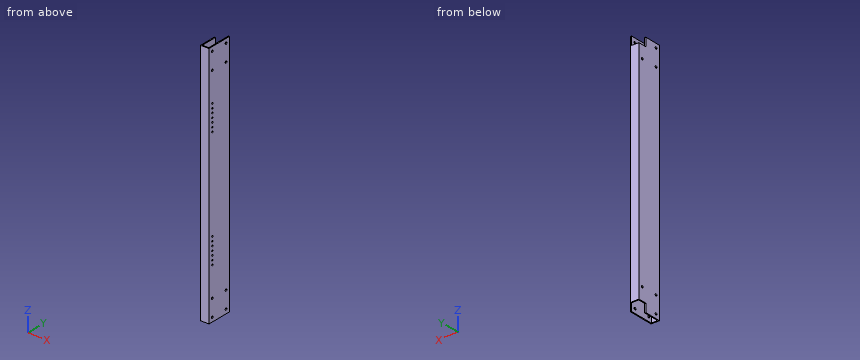
```python
from build123d import *

# Parameters (mm, degrees)
SKETCH1_W               = 25.4
SKETCH1_H               = 76.2
BOSS_EXTRUDE1_DEPTH     = 368.3
SHELL1_T                = -3.175
CUT_EXTRUDE2_REACH      = 27.4
SKETCH3_R               = 2.38125
SKETCH4_W               = 25.4
SKETCH4_H               = 25.4
CUT_EXTRUDE3_DEPTH      = 22.225
SKETCH5_R               = 3.25
CUT_EXTRUDE4_DEPTH      = 23.225
CUT_EXTRUDE4_DEPTH_BACK = 4.175


with BuildPart() as part:
    # Sketch1 → Boss-Extrude1 (new body, symmetric)
    with BuildSketch(Plane.XY):
        Rectangle(SKETCH1_W, SKETCH1_H)
    extrude(amount=BOSS_EXTRUDE1_DEPTH, both=True)

    # Shell1
    shell1_openings = [part.faces().sort_by_distance(p)[0] for p in [
        (0, 0, 368.3),
        (0, 0, -368.3),
    ]]
    offset(amount=SHELL1_T, openings=shell1_openings, kind=Kind.INTERSECTION)

    # Sketch3 → Cut-Extrude2 (cut, up to next)
    with BuildSketch(Plane(origin=(12.7, 0, 0), x_dir=(0, 0, -1), z_dir=(1, 0, 0)), mode=Mode.PRIVATE) as cut_extrude2_sk1:
        with Locations((215.9, -25.4)):
            Circle(SKETCH3_R)
    cut_extrude2_tool1 = extrude(cut_extrude2_sk1.sketch, amount=-CUT_EXTRUDE2_REACH, mode=Mode.PRIVATE) & part.part
    add(cut_extrude2_tool1.solids().sort_by_distance((12.7, -25.4, -215.9))[0], mode=Mode.SUBTRACT)
    # Sketch3 → Cut-Extrude2 (cut, up to next)
    with BuildSketch(Plane(origin=(12.7, 0, 0), x_dir=(0, 0, -1), z_dir=(1, 0, 0)), mode=Mode.PRIVATE) as cut_extrude2_sk2:
        with Locations((203.2, -25.4)):
            Circle(SKETCH3_R)
    cut_extrude2_tool2 = extrude(cut_extrude2_sk2.sketch, amount=-CUT_EXTRUDE2_REACH, mode=Mode.PRIVATE) & part.part
    add(cut_extrude2_tool2.solids().sort_by_distance((12.7, -25.4, -203.2))[0], mode=Mode.SUBTRACT)
    # Sketch3 → Cut-Extrude2 (cut, up to next)
    with BuildSketch(Plane(origin=(12.7, 0, 0), x_dir=(0, 0, -1), z_dir=(1, 0, 0)), mode=Mode.PRIVATE) as cut_extrude2_sk3:
        with Locations((190.5, -25.4)):
            Circle(SKETCH3_R)
    cut_extrude2_tool3 = extrude(cut_extrude2_sk3.sketch, amount=-CUT_EXTRUDE2_REACH, mode=Mode.PRIVATE) & part.part
    add(cut_extrude2_tool3.solids().sort_by_distance((12.7, -25.4, -190.5))[0], mode=Mode.SUBTRACT)
    # Sketch3 → Cut-Extrude2 (cut, up to next)
    with BuildSketch(Plane(origin=(12.7, 0, 0), x_dir=(0, 0, -1), z_dir=(1, 0, 0)), mode=Mode.PRIVATE) as cut_extrude2_sk4:
        with Locations((177.8, -25.4)):
            Circle(SKETCH3_R)
    cut_extrude2_tool4 = extrude(cut_extrude2_sk4.sketch, amount=-CUT_EXTRUDE2_REACH, mode=Mode.PRIVATE) & part.part
    add(cut_extrude2_tool4.solids().sort_by_distance((12.7, -25.4, -177.8))[0], mode=Mode.SUBTRACT)
    # Sketch3 → Cut-Extrude2 (cut, up to next)
    with BuildSketch(Plane(origin=(12.7, 0, 0), x_dir=(0, 0, -1), z_dir=(1, 0, 0)), mode=Mode.PRIVATE) as cut_extrude2_sk5:
        with Locations((165.1, -25.4)):
            Circle(SKETCH3_R)
    cut_extrude2_tool5 = extrude(cut_extrude2_sk5.sketch, amount=-CUT_EXTRUDE2_REACH, mode=Mode.PRIVATE) & part.part
    add(cut_extrude2_tool5.solids().sort_by_distance((12.7, -25.4, -165.1))[0], mode=Mode.SUBTRACT)
    # Sketch3 → Cut-Extrude2 (cut, up to next)
    with BuildSketch(Plane(origin=(12.7, 0, 0), x_dir=(0, 0, -1), z_dir=(1, 0, 0)), mode=Mode.PRIVATE) as cut_extrude2_sk6:
        with Locations((152.4, -25.4)):
            Circle(SKETCH3_R)
    cut_extrude2_tool6 = extrude(cut_extrude2_sk6.sketch, amount=-CUT_EXTRUDE2_REACH, mode=Mode.PRIVATE) & part.part
    add(cut_extrude2_tool6.solids().sort_by_distance((12.7, -25.4, -152.4))[0], mode=Mode.SUBTRACT)
    # Sketch3 → Cut-Extrude2 (cut, up to next)
    with BuildSketch(Plane(origin=(12.7, 0, 0), x_dir=(0, 0, -1), z_dir=(1, 0, 0)), mode=Mode.PRIVATE) as cut_extrude2_sk7:
        with Locations((139.7, -25.4)):
            Circle(SKETCH3_R)
    cut_extrude2_tool7 = extrude(cut_extrude2_sk7.sketch, amount=-CUT_EXTRUDE2_REACH, mode=Mode.PRIVATE) & part.part
    add(cut_extrude2_tool7.solids().sort_by_distance((12.7, -25.4, -139.7))[0], mode=Mode.SUBTRACT)
    # Sketch3 → Cut-Extrude2 (cut, up to next)
    with BuildSketch(Plane(origin=(12.7, 0, 0), x_dir=(0, 0, -1), z_dir=(1, 0, 0)), mode=Mode.PRIVATE) as cut_extrude2_sk8:
        with Locations((-139.7, -25.4)):
            Circle(SKETCH3_R)
    cut_extrude2_tool8 = extrude(cut_extrude2_sk8.sketch, amount=-CUT_EXTRUDE2_REACH, mode=Mode.PRIVATE) & part.part
    add(cut_extrude2_tool8.solids().sort_by_distance((12.7, -25.4, 139.7))[0], mode=Mode.SUBTRACT)
    # Sketch3 → Cut-Extrude2 (cut, up to next)
    with BuildSketch(Plane(origin=(12.7, 0, 0), x_dir=(0, 0, -1), z_dir=(1, 0, 0)), mode=Mode.PRIVATE) as cut_extrude2_sk9:
        with Locations((-152.4, -25.4)):
            Circle(SKETCH3_R)
    cut_extrude2_tool9 = extrude(cut_extrude2_sk9.sketch, amount=-CUT_EXTRUDE2_REACH, mode=Mode.PRIVATE) & part.part
    add(cut_extrude2_tool9.solids().sort_by_distance((12.7, -25.4, 152.4))[0], mode=Mode.SUBTRACT)
    # Sketch3 → Cut-Extrude2 (cut, up to next)
    with BuildSketch(Plane(origin=(12.7, 0, 0), x_dir=(0, 0, -1), z_dir=(1, 0, 0)), mode=Mode.PRIVATE) as cut_extrude2_sk10:
        with Locations((-165.1, -25.4)):
            Circle(SKETCH3_R)
    cut_extrude2_tool10 = extrude(cut_extrude2_sk10.sketch, amount=-CUT_EXTRUDE2_REACH, mode=Mode.PRIVATE) & part.part
    add(cut_extrude2_tool10.solids().sort_by_distance((12.7, -25.4, 165.1))[0], mode=Mode.SUBTRACT)
    # Sketch3 → Cut-Extrude2 (cut, up to next)
    with BuildSketch(Plane(origin=(12.7, 0, 0), x_dir=(0, 0, -1), z_dir=(1, 0, 0)), mode=Mode.PRIVATE) as cut_extrude2_sk11:
        with Locations((-203.2, -25.4)):
            Circle(SKETCH3_R)
    cut_extrude2_tool11 = extrude(cut_extrude2_sk11.sketch, amount=-CUT_EXTRUDE2_REACH, mode=Mode.PRIVATE) & part.part
    add(cut_extrude2_tool11.solids().sort_by_distance((12.7, -25.4, 203.2))[0], mode=Mode.SUBTRACT)
    # Sketch3 → Cut-Extrude2 (cut, up to next)
    with BuildSketch(Plane(origin=(12.7, 0, 0), x_dir=(0, 0, -1), z_dir=(1, 0, 0)), mode=Mode.PRIVATE) as cut_extrude2_sk12:
        with Locations((-177.8, -25.4)):
            Circle(SKETCH3_R)
    cut_extrude2_tool12 = extrude(cut_extrude2_sk12.sketch, amount=-CUT_EXTRUDE2_REACH, mode=Mode.PRIVATE) & part.part
    add(cut_extrude2_tool12.solids().sort_by_distance((12.7, -25.4, 177.8))[0], mode=Mode.SUBTRACT)
    # Sketch3 → Cut-Extrude2 (cut, up to next)
    with BuildSketch(Plane(origin=(12.7, 0, 0), x_dir=(0, 0, -1), z_dir=(1, 0, 0)), mode=Mode.PRIVATE) as cut_extrude2_sk13:
        with Locations((-215.9, -25.4)):
            Circle(SKETCH3_R)
    cut_extrude2_tool13 = extrude(cut_extrude2_sk13.sketch, amount=-CUT_EXTRUDE2_REACH, mode=Mode.PRIVATE) & part.part
    add(cut_extrude2_tool13.solids().sort_by_distance((12.7, -25.4, 215.9))[0], mode=Mode.SUBTRACT)
    # Sketch3 → Cut-Extrude2 (cut, up to next)
    with BuildSketch(Plane(origin=(12.7, 0, 0), x_dir=(0, 0, -1), z_dir=(1, 0, 0)), mode=Mode.PRIVATE) as cut_extrude2_sk14:
        with Locations((-190.5, -25.4)):
            Circle(SKETCH3_R)
    cut_extrude2_tool14 = extrude(cut_extrude2_sk14.sketch, amount=-CUT_EXTRUDE2_REACH, mode=Mode.PRIVATE) & part.part
    add(cut_extrude2_tool14.solids().sort_by_distance((12.7, -25.4, 190.5))[0], mode=Mode.SUBTRACT)

    # Sketch4 → Cut-Extrude3 (cut)
    with BuildSketch(Plane.ZY.offset(12.7)):
        with Locations((-355.6, 25.4)):
            Rectangle(SKETCH4_W, SKETCH4_H)
        with Locations((355.6, 25.4)):
            Rectangle(SKETCH4_W, SKETCH4_H)
    extrude(amount=-CUT_EXTRUDE3_DEPTH, mode=Mode.SUBTRACT)

    # Sketch5 → Cut-Extrude4 (cut, two sides)
    with BuildSketch(Plane.ZY.offset(-9.525)) as cut_extrude4_sk:
        with Locations((-355.6, 25.4)):
            Circle(SKETCH5_R)
        with Locations((355.6, 25.4)):
            Circle(SKETCH5_R)
        with Locations((-355.6, -25.4)):
            Circle(SKETCH5_R)
        with Locations((-304.8, -25.4)):
            Circle(SKETCH5_R)
        with Locations((-304.8, 25.4)):
            Circle(SKETCH5_R)
        with Locations((304.8, 25.4)):
            Circle(SKETCH5_R)
        with Locations((304.8, -25.4)):
            Circle(SKETCH5_R)
        with Locations((355.6, -25.4)):
            Circle(SKETCH5_R)
    extrude(amount=CUT_EXTRUDE4_DEPTH, mode=Mode.SUBTRACT)
    extrude(cut_extrude4_sk.sketch, amount=-CUT_EXTRUDE4_DEPTH_BACK, mode=Mode.SUBTRACT)


solid = part.part
```
Can you work these out from the model? Positions are in its coordinate system, mm. Coordinates: 2 decimals unless noted, no trailing zeros. Write each loop counter-clockwise with the first axis right and the second up, starting at its lowest first coordinate (ties: lowest second). Pieces come first, ordered by that corner, then holes. Notation, with made-up numbers: (34.5, 57) - (71.5, 57) arc R35 cw to (71.5, 90) - close; hole circle Ø6 at (67, -29.75). An arc over 180 degrees is marked (long way). Return JSON: item names as keys, results as strings.
Q1. If we section it at B-B (z = -237): Please give me the cut outline in (x, y) (3 decimals).
Computed values:
{"outline": "(-12.7, -38.1) - (12.7, -38.1) - (12.7, 38.1) - (-12.7, 38.1) - close; hole (-9.525, -34.925) - (9.525, -34.925) - (9.525, 34.925) - (-9.525, 34.925) - close"}
Q2. I'm going to push flat-ended pins straight in: pin 1 Ø4.5 at (y, z) = (-25.4, 177.8) entering from +X (3 decimals); pin 2 Ø10 at (x, y) = (-0.5, -24) entering from -Z; pin 3 Ø11 at (x, y) = (3.5, 31.5) entering from -Z. Where does each tip first touch, or does it pass through?
Computed values:
{"pin 1": "stops at x = -9.525", "pin 2": "passes through", "pin 3": "stops at z = -342.9"}
Q3. If we section it at C-C (x = 0.75): Please give me the cut outline in (y, z) (3 decimals), then the cut area to 3 significant figures.
Computed values:
{"outline": "(-38.1, -368.3) - (-34.925, -368.3) - (-34.925, 368.3) - (-38.1, 368.3) - close; (34.925, -342.9) - (38.1, -342.9) - (38.1, 342.9) - (34.925, 342.9) - close", "area": "4,520 mm2"}
Q4. Please list where these lines run through material, in increasing order: L1, parallel to Z at x = -10.8, y = 25.4; L2, parallel to Y at x = 3, z = 130.5 (3 decimals); L3, parallel to X at y = 11, z = 317 (3 decimals). Write a range as from..to.
Computed values:
{"L1": "z = -342.9..-308.05, -301.55..301.55, 308.05..342.9", "L2": "y = -38.1..-34.925, 34.925..38.1", "L3": "x = -12.7..-9.525, 9.525..12.7"}
Q5. If we section it at A-A (y = -4): Please give me the cut outline in (x, z) (3 decimals), then the cut area to 3 significant figures.
Computed values:
{"outline": "(-12.7, -368.3) - (-9.525, -368.3) - (-9.525, 368.3) - (-12.7, 368.3) - close; (9.525, -368.3) - (12.7, -368.3) - (12.7, 368.3) - (9.525, 368.3) - close", "area": "4,680 mm2"}
